Read the model definition and answer for the solid it produces. Units are mm, in the model's axes. Coordinates: 2 decimals unless noted, no trailing zeros. Loops run counter-clockwise (first coordinate to the right, second up) from the corner with the lowest first, then second, coordinate; pieces in that order, holes last.
from build123d import *

# Parameters (mm, degrees)
SKETCH_1_R          = 75
EXTRUDE_1_DEPTH     = 8
FILLET_1_R          = 7
FILLET_2_R          = 7
FILLET_3_R          = 7
SKETCH_2_R          = 5
CUT_EXTRUDE_1_DEPTH = 10
SKETCH_3_R          = 1.5
CUT_EXTRUDE_2_DEPTH = 10
FILLET_4_R          = 7


with BuildPart() as part:
    # 草图1 → 凸台-拉伸1 (new body)
    with BuildSketch(Plane(origin=(0, 0, 0), x_dir=(1, 0, 0), z_dir=(0, 1, 0))):
        with Locations(Location((0, 0, 0), (0, 0, 270))):
            Circle(SKETCH_1_R)
        with BuildLine():
            Line((-5.48403898, -21.821441668), (-6.099248264, -49.626597411))
            ThreePointArc((-6.099248264, -49.626597411), (-43.843682887, -24.036045242), (-45.11861404, 21.547869201))
            Line((-45.11861404, 21.547869201), (-21.346247453, 7.11250446))
            ThreePointArc((-21.346247453, 7.11250446), (-19.729657299, -10.816220359), (-5.48403898, -21.821441668))
        make_face(mode=Mode.SUBTRACT)
        with BuildLine():
            Line((-39.928269929, 30.095402646), (-16.155903342, 15.660037906))
            ThreePointArc((-16.155903342, 15.660037906), (0.497707046, 22.494494609), (16.832733273, 14.930140339))
            Line((16.832733273, 14.930140339), (41.220309145, 28.299931342))
            ThreePointArc((41.220309145, 28.299931342), (1.106015658, 49.987765797), (-39.928269929, 30.095402646))
        make_face(mode=Mode.SUBTRACT)
        with BuildLine():
            Line((4.513514179, -22.042644799), (3.898304895, -49.847800543))
            ThreePointArc((3.898304895, -49.847800543), (42.73766723, -25.951720555), (46.027518194, 19.531194765))
            Line((46.027518194, 19.531194765), (21.639942322, 6.161403762))
            ThreePointArc((21.639942322, 6.161403762), (19.231950253, -11.67827425), (4.513514179, -22.042644799))
        make_face(mode=Mode.SUBTRACT)
    extrude(amount=EXTRUDE_1_DEPTH)

    # 圆角1
    fillet_1_edges = [part.edges().sort_by_distance(p)[0] for p in [
        (41.220309145, 4, -28.299931342),
    ]]
    fillet(fillet_1_edges, radius=FILLET_1_R)

    # 圆角2
    fillet_2_edges = [part.edges().sort_by_distance(p)[0] for p in [
        (-39.928269929, 4, -30.095402646),
    ]]
    fillet(fillet_2_edges, radius=FILLET_2_R)

    # 圆角3
    fillet_3_edges = [part.edges().sort_by_distance(p)[0] for p in [
        (3.898304895, 4, 49.847800543),
        (46.027518194, 4, -19.531194765),
        (-45.11861404, 4, -21.547869201),
        (-6.099248264, 4, 49.626597411),
    ]]
    fillet(fillet_3_edges, radius=FILLET_3_R)

    # 草图2 → 切除-拉伸1 (cut)
    with BuildSketch(Plane(origin=(0, 8, 0), x_dir=(1, 0, 0), z_dir=(0, 1, 0))):
        with Locations(Location((0, 0, 0), (0, 0, 270))):
            Circle(SKETCH_2_R)
    extrude(amount=-CUT_EXTRUDE_1_DEPTH, mode=Mode.SUBTRACT)

    # 草图3 → 切除-拉伸2 (cut)
    with BuildSketch(Plane(origin=(0, 8, 0), x_dir=(1, 0, 0), z_dir=(0, 1, 0))):
        with Locations(Location((-13.248676841, 8.045033372, 0), (0, 0, 270))):
            Circle(SKETCH_3_R)
        with Locations(Location((8.045033372, 13.248676841, 0), (0, 0, 270))):
            Circle(SKETCH_3_R)
        with Locations(Location((13.248676841, -8.045033372, 0), (0, 0, 270))):
            Circle(SKETCH_3_R)
        with Locations(Location((-8.045033372, -13.248676841, 0), (0, 0, 270))):
            Circle(SKETCH_3_R)
    extrude(amount=-CUT_EXTRUDE_2_DEPTH, mode=Mode.SUBTRACT)

    # 圆角4
    fillet_4_edges = [part.edges().sort_by_distance(p)[0] for p in [
        (-16.155903342, 4, -15.660037906),
        (16.832733273, 4, -14.930140339),
        (21.639942322, 4, -6.161403762),
        (4.513514179, 4, 22.042644799),
        (-5.48403898, 4, 21.821441668),
        (-21.346247453, 4, -7.11250446),
    ]]
    fillet(fillet_4_edges, radius=FILLET_4_R)


solid = part.part
Item 1: Given pin 1 (2.5 mm diameter, centred on x = 13.25, z = 8.05, fed in from +Y); pin 2 (4 mm diameter, centred on x = 19, y = 6, fed in from +Z); pin 3 (4 mm diameter, centred on x = -13.25, z = -8.05, fed in from -Y); pin 4 (1 mm diameter, centred on y = 7, z = 33.5, fed in from +X), each flat-ended and moving along its own axis, determine where each tip first touches the part or whether it passes through.
Numbers:
pin 1: passes through
pin 2: stops at z = 73.05
pin 3: stops at y = 0
pin 4: stops at x = 67.35
Item 2: A cutting plane is placed at B-B on z = 0. Determine the outline of the cut face in (x, y).
Numbers:
outline: (-75, 0) - (-50, 0) - (-50, 8) - (-75, 8) - close; (-22.5, 0) - (-5, 0) - (-5, 8) - (-22.5, 8) - close; (5, 0) - (22.5, 0) - (22.5, 8) - (5, 8) - close; (50, 0) - (75, 0) - (75, 8) - (50, 8) - close
Item 3: Find the intervals of material crossed by line 1 along X through (y, z) = (5.5, 0); line 2 along X through (y, z) = (3.75, -10.5); line 3 along Z through (x, y) = (-17, 7.75), in increasing order.
Numbers:
line 1: x = -75 to -50, -22.5 to -5, 5 to 22.5, 50 to 75
line 2: x = -74.26 to -48.89, -26.92 to 29.55, 48.89 to 74.26
line 3: z = -73.05 to -47.02, -17.25 to 14.74, 47.02 to 73.05
Item 4: A cutting plane is placed at C-C on y = 3.5. Give the number of separate pieces and of enclosed holes in the cut face, then the cut area to 3 significant figures.
Numbers:
separate pieces: 1
enclosed holes: 8
area: 12,300 mm2
Item 5: A cutting plane is placed at D-D on x = 28. Determine the outline of the cut face in (y, z), then the cut area to 3 significant figures.
Numbers:
outline: (0, -69.58) - (8, -69.58) - (8, -41.42) - (0, -41.42) - close; (0, -21.05) - (8, -21.05) - (8, -9.65) - (0, -9.65) - close; (0, 41.42) - (8, 41.42) - (8, 69.58) - (0, 69.58) - close
area: 542 mm2
Item 6: Determine the mould class of faces 1 (the face through (37.38, 4.06, -29.47)), 2 (the face through (1, 8, 16)) for opening direction X: released by +X, released by -X, zero draft, split by the parting line, or undercut.
Numbers:
face 1: undercut
face 2: zero draft
Item 7: A cutting plane is placed at A-A on x = 0. Determine the outline of the cut face in (y, z).
Numbers:
outline: (0, -75) - (8, -75) - (8, -50) - (0, -50) - close; (0, -22.5) - (8, -22.5) - (8, -5) - (0, -5) - close; (0, 5) - (8, 5) - (8, 75) - (0, 75) - close
